Could you check a few things on this drawing? It's one solid part, dimensions in mm from its lowest x, y, z. Round coordinates to 2 decimals unless told otherwise and drop trailing zeros. Write each loop counter-clockwise with the first axis right and the second up, starting at its lowest first coordinate (ties: lowest second). Pieces come first, ordered by that corner, then holes. Notation, with made-up numbers: (-18.5, -31.75) -> (11.5, -31.75) arc R30 ccw to (11.5, -7.75) -> close; hole circle Ø6 at (30, 59.5). An arc over 180 degrees is marked (long way). Return JSON: item names as keys, results as strings.
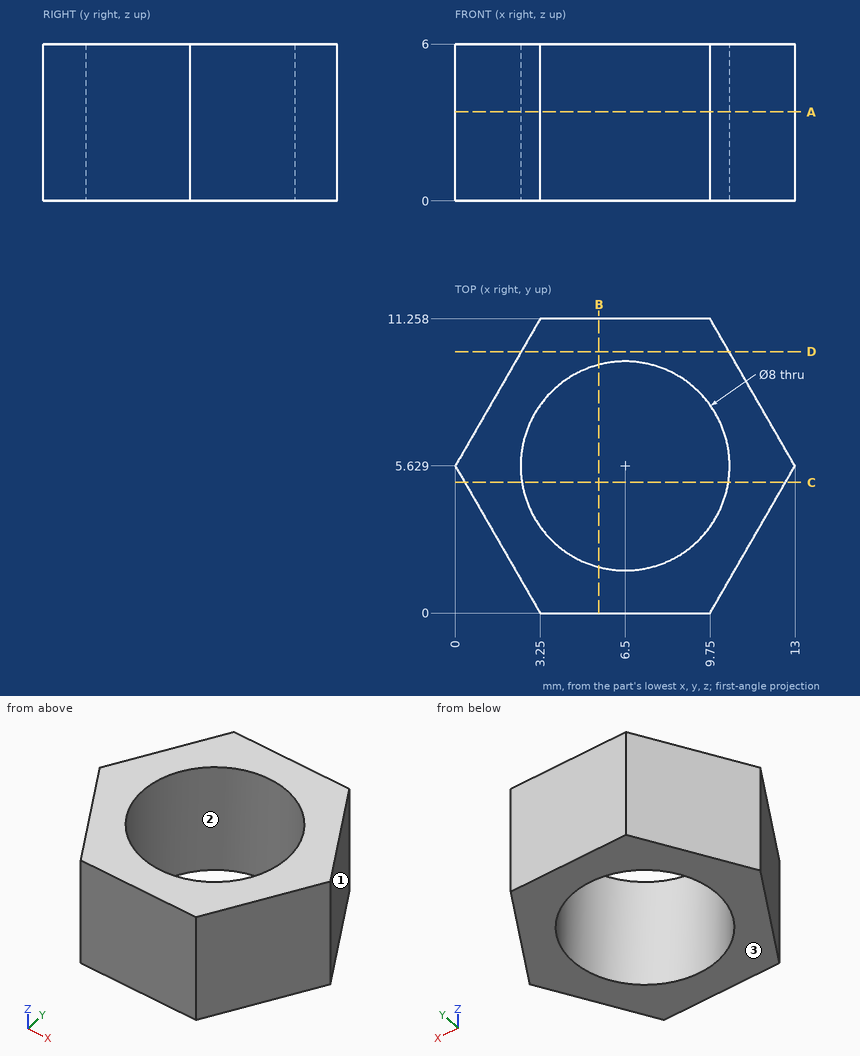
1) If I drill on probe 1 along Y at (x, z) = (6.5, 4.5); probe 2 along X at (y, z) = (5, 2.8); probe 3 along Y at (x, z) = (4.5, 5.65) (1 decimal), over which ranges is the centre line in solid material (lowest first)? Write a range as [from, to].
Return value:
{"probe 1": "[0, 1.63], [9.63, 11.26]", "probe 2": "[0.36, 2.55], [10.45, 12.64]", "probe 3": "[0, 2.2], [9.1, 11.3]"}
2) Will these pins go through, and if not, where does the flat tip stop? pin 1 Ø1 at (y, z) = (9.5, 5) entering from -X; pin 2 Ø1 at (x, z) = (1.5, 3) entering from +Y (1 decimal).
Return value:
{"pin 1": "x = 1.95", "pin 2": "y = 9.1"}
3) I want a section at A-A, the plane z = 3.4. Please give me the cut outline in (x, y).
Return value:
{"outline": "(0, 5.63) -> (3.25, 0) -> (9.75, 0) -> (13, 5.63) -> (9.75, 11.26) -> (3.25, 11.26) -> close; hole circle Ø8 at (6.5, 5.63)"}
4) Thinking about a two-plate mould opening in X: for the marked faces 1, 2 and 3, which applies, pulls with the +X half, pulls with the -X half, needs draft (parallel to the pull), parting line crosses it, or undercut?
Return value:
{"face 1": "pulls with the +X half", "face 2": "undercut", "face 3": "needs draft"}
5) I want a section at D-D, the plane y = 10. Please give me the cut outline in (x, z).
Return value:
{"outline": "(2.52, 0) -> (10.48, 0) -> (10.48, 6) -> (2.52, 6) -> close"}
6) I want a section at B-B, the plane x = 5.5. Please give me the cut outline in (y, z), and give its area (3 significant figures).
Return value:
{"outline": "(0, 0) -> (1.76, 0) -> (1.76, 6) -> (0, 6) -> close; (9.5, 0) -> (11.26, 0) -> (11.26, 6) -> (9.5, 6) -> close", "area": "21.1 mm²"}
7) I want a section at C-C, the plane y = 5. Please give me the cut outline in (x, z).
Return value:
{"outline": "(0.36, 0) -> (2.55, 0) -> (2.55, 6) -> (0.36, 6) -> close; (10.45, 0) -> (12.64, 0) -> (12.64, 6) -> (10.45, 6) -> close"}
